Input: part model. Units: mm. Frame: model coordinates. A direction names the side the tool comes from. Coordinates: 2 decimals unless noted, no trailing zeros. Write each loop counter-clockwise with the first axis right and the second up, starting at its lowest first coordinate (ties: lowest second). Pieces come first, ordered by that corner, then holes. Notation, with made-up numbers: M 11.5,45.25 L 29.5,45.25 A18 ccw 29.5,58.25 Z; hole C 55,84.5 d7. An arc over 180 degrees is marked long. Use one line per item in the form item = value.
from build123d import *
from OCP.BRepFilletAPI import BRepFilletAPI_MakeChamfer

# Parameters (mm, degrees)
SKETCH_1_R          = 10
EXTRUDE_1_DEPTH     = 2
SKETCH_2_R          = 10
SKETCH_2_R_2        = 8.5
EXTRUDE_2_DEPTH     = 3
SKETCH_4_R          = 13.5
SKETCH_4_R_2        = 8.5
EXTRUDE_3_DEPTH     = 1
SKETCH_5_R          = 12.25
SKETCH_5_R_2        = 8.5
EXTRUDE_4_DEPTH     = 8
SKETCH_6_R          = 0.9
CUT_EXTRUDE_1_DEPTH = 8
SKETCH_7_R          = 3
SKETCH_7_R_2        = 1.15
CUT_EXTRUDE_2_DEPTH = 24.674881204
SKETCH_9_W          = 3
SKETCH_9_H          = 17
CUT_EXTRUDE_4_DEPTH = 24.674881204
EXTRUDE_5_DEPTH     = 3
CHAMFER_1_SIZE      = 0.2
CHAMFER_1_SIZE2     = 0.410060768


with BuildPart() as part:
    # 스케치1 → 보스-돌출1 (new body)
    with BuildSketch(Plane.XY):
        Circle(SKETCH_1_R)
    extrude(amount=EXTRUDE_1_DEPTH)

    # 스케치2 → 보스-돌출2 (add)
    with BuildSketch(Plane.XY.offset(2)):
        Circle(SKETCH_2_R)
        Circle(SKETCH_2_R_2, mode=Mode.SUBTRACT)
    extrude(amount=EXTRUDE_2_DEPTH)

    # 스케치4 → 보스-돌출3 (add)
    with BuildSketch(Plane.XY.offset(5)):
        Circle(SKETCH_4_R)
        Circle(SKETCH_4_R_2, mode=Mode.SUBTRACT)
    extrude(amount=EXTRUDE_3_DEPTH)

    # 스케치5 → 보스-돌출4 (add)
    with BuildSketch(Plane.XY.offset(6)):
        Circle(SKETCH_5_R)
        Circle(SKETCH_5_R_2, mode=Mode.SUBTRACT)
    extrude(amount=EXTRUDE_4_DEPTH)

    # 스케치6 → 컷-돌출1 (cut)
    with BuildSketch(Plane.XY.offset(14)):
        with Locations((10.375, 0)):
            Circle(SKETCH_6_R)
        with Locations((5.1875, -8.985013564)):
            Circle(SKETCH_6_R)
        with Locations((-5.1875, -8.985013564)):
            Circle(SKETCH_6_R)
        with Locations((-10.375, 0)):
            Circle(SKETCH_6_R)
        with Locations((-5.1875, 8.985013564)):
            Circle(SKETCH_6_R)
        with Locations((5.1875, 8.985013564)):
            Circle(SKETCH_6_R)
    extrude(amount=-CUT_EXTRUDE_1_DEPTH, mode=Mode.SUBTRACT)

    # 스케치7 → 컷-돌출2 (cut, through all)
    with BuildSketch(Plane(origin=(0, 0, 0), x_dir=(-1, 0, 0), z_dir=(0, 0, -1))):
        Circle(SKETCH_7_R)
        with Locations((-7, 0)):
            Circle(SKETCH_7_R_2)
        with Locations((7, 0)):
            Circle(SKETCH_7_R_2)
        with Locations((0, 7)):
            Circle(SKETCH_7_R_2)
        with Locations((0, -7)):
            Circle(SKETCH_7_R_2)
    extrude(amount=-CUT_EXTRUDE_2_DEPTH, mode=Mode.SUBTRACT)

    # 스케치9 → 컷-돌출4 (cut, through all)
    with BuildSketch(Plane(origin=(0, 0, 0), x_dir=(0, 0, -1), z_dir=(1, 0, 0))):
        with Locations((-3.5, 0)):
            Rectangle(SKETCH_9_W, SKETCH_9_H)
    extrude(amount=-CUT_EXTRUDE_4_DEPTH, mode=Mode.SUBTRACT)

    # 스케치10 → 보스-돌출5 (add)
    with BuildSketch(Plane.XY.offset(14)):
        with BuildLine():
            Line((2.199961883, 8.210369523), (2.717599974, 10.142221176))
            ThreePointArc((2.717599974, 10.142221176), (0, 10.5), (-2.717599974, 10.142221176))
            Line((-2.717599974, 10.142221176), (-2.199961883, 8.210369523))
            ThreePointArc((-2.199961883, 8.210369523), (0, 8.5), (2.199961883, 8.210369523))
        make_face()
        with BuildLine():
            Line((6.01040764, 6.01040764), (7.424621202, 7.424621202))
            ThreePointArc((7.424621202, 7.424621202), (9.09326674, 5.25), (10.142221176, 2.717599974))
            Line((10.142221176, 2.717599974), (8.210369523, 2.199961883))
            ThreePointArc((8.210369523, 2.199961883), (7.361215932, 4.25), (6.01040764, 6.01040764))
        make_face()
        with BuildLine():
            Line((8.210369523, -2.199961883), (10.142221176, -2.717599974))
            ThreePointArc((10.142221176, -2.717599974), (9.09326674, -5.25), (7.424621202, -7.424621202))
            Line((7.424621202, -7.424621202), (6.01040764, -6.01040764))
            ThreePointArc((6.01040764, -6.01040764), (7.361215932, -4.25), (8.210369523, -2.199961883))
        make_face()
        with BuildLine():
            Line((2.199961883, -8.210369523), (2.717599974, -10.142221176))
            ThreePointArc((2.717599974, -10.142221176), (0, -10.5), (-2.717599974, -10.142221176))
            Line((-2.717599974, -10.142221176), (-2.199961883, -8.210369523))
            ThreePointArc((-2.199961883, -8.210369523), (0, -8.5), (2.199961883, -8.210369523))
        make_face()
        with BuildLine():
            Line((-6.01040764, -6.01040764), (-7.424621202, -7.424621202))
            ThreePointArc((-7.424621202, -7.424621202), (-9.09326674, -5.25), (-10.142221176, -2.717599974))
            Line((-10.142221176, -2.717599974), (-8.210369523, -2.199961883))
            ThreePointArc((-8.210369523, -2.199961883), (-7.361215932, -4.25), (-6.01040764, -6.01040764))
        make_face()
        with BuildLine():
            Line((-8.210369523, 2.199961883), (-10.142221176, 2.717599974))
            ThreePointArc((-10.142221176, 2.717599974), (-9.09326674, 5.25), (-7.424621202, 7.424621202))
            Line((-7.424621202, 7.424621202), (-6.01040764, 6.01040764))
            ThreePointArc((-6.01040764, 6.01040764), (-7.361215932, 4.25), (-8.210369523, 2.199961883))
        make_face()
    extrude(amount=EXTRUDE_5_DEPTH)

    # 모따기1: one chamfer whose edges measure the first distance from different faces: ONE call of the kernel's chamfer builder (chamfer() names one face for all edges)
    chamfer_1_edges_1 = [part.edges().sort_by_distance(p)[0] for p in [
        (-6.717514421, 6.717514421, 17),
    ]]
    chamfer_1_side_1 = [part.faces().sort_by_distance(p)[0] for p in [
        (-6.717514421, 6.717514421, 15.5),
    ]]
    chamfer_1_edges_2 = [part.edges().sort_by_distance(p)[0] for p in [
        (-9.09326674, 5.25, 17),
    ]]
    chamfer_1_side_2 = [part.faces().sort_by_distance(p)[0] for p in [
        (-9.09326674, 5.25, 15.5),
    ]]
    chamfer_1_edges_3 = [part.edges().sort_by_distance(p)[0] for p in [
        (-9.17629535, 2.458780928, 17),
    ]]
    chamfer_1_side_3 = [part.faces().sort_by_distance(p)[0] for p in [
        (-9.17629535, 2.458780928, 15.5),
    ]]
    chamfer_1_edges_4 = [part.edges().sort_by_distance(p)[0] for p in [
        (-9.17629535, -2.458780928, 17),
    ]]
    chamfer_1_side_4 = [part.faces().sort_by_distance(p)[0] for p in [
        (-9.17629535, -2.458780928, 15.5),
    ]]
    chamfer_1_edges_5 = [part.edges().sort_by_distance(p)[0] for p in [
        (-9.09326674, -5.25, 17),
    ]]
    chamfer_1_side_5 = [part.faces().sort_by_distance(p)[0] for p in [
        (-9.09326674, -5.25, 15.5),
    ]]
    chamfer_1_edges_6 = [part.edges().sort_by_distance(p)[0] for p in [
        (-6.717514421, -6.717514421, 17),
    ]]
    chamfer_1_side_6 = [part.faces().sort_by_distance(p)[0] for p in [
        (-6.717514421, -6.717514421, 15.5),
    ]]
    chamfer_1_edges_7 = [part.edges().sort_by_distance(p)[0] for p in [
        (0, 10.5, 17),
    ]]
    chamfer_1_side_7 = [part.faces().sort_by_distance(p)[0] for p in [
        (0, 10.5, 15.5),
    ]]
    chamfer_1_edges_8 = [part.edges().sort_by_distance(p)[0] for p in [
        (-2.458780928, 9.17629535, 17),
    ]]
    chamfer_1_side_8 = [part.faces().sort_by_distance(p)[0] for p in [
        (-2.458780928, 9.17629535, 15.5),
    ]]
    chamfer_1_edges_9 = [part.edges().sort_by_distance(p)[0] for p in [
        (2.458780928, 9.17629535, 17),
    ]]
    chamfer_1_side_9 = [part.faces().sort_by_distance(p)[0] for p in [
        (2.458780928, 9.17629535, 15.5),
    ]]
    chamfer_1_edges_10 = [part.edges().sort_by_distance(p)[0] for p in [
        (-2.458780928, -9.17629535, 17),
    ]]
    chamfer_1_side_10 = [part.faces().sort_by_distance(p)[0] for p in [
        (-2.458780928, -9.17629535, 15.5),
    ]]
    chamfer_1_edges_11 = [part.edges().sort_by_distance(p)[0] for p in [
        (0, -10.5, 17),
    ]]
    chamfer_1_side_11 = [part.faces().sort_by_distance(p)[0] for p in [
        (0, -10.5, 15.5),
    ]]
    chamfer_1_edges_12 = [part.edges().sort_by_distance(p)[0] for p in [
        (2.458780928, -9.17629535, 17),
    ]]
    chamfer_1_side_12 = [part.faces().sort_by_distance(p)[0] for p in [
        (2.458780928, -9.17629535, 15.5),
    ]]
    chamfer_1_edges_13 = [part.edges().sort_by_distance(p)[0] for p in [
        (9.09326674, 5.25, 17),
    ]]
    chamfer_1_side_13 = [part.faces().sort_by_distance(p)[0] for p in [
        (9.09326674, 5.25, 15.5),
    ]]
    chamfer_1_edges_14 = [part.edges().sort_by_distance(p)[0] for p in [
        (6.717514421, 6.717514421, 17),
    ]]
    chamfer_1_side_14 = [part.faces().sort_by_distance(p)[0] for p in [
        (6.717514421, 6.717514421, 15.5),
    ]]
    chamfer_1_edges_15 = [part.edges().sort_by_distance(p)[0] for p in [
        (9.17629535, 2.458780928, 17),
    ]]
    chamfer_1_side_15 = [part.faces().sort_by_distance(p)[0] for p in [
        (9.17629535, 2.458780928, 15.5),
    ]]
    chamfer_1_edges_16 = [part.edges().sort_by_distance(p)[0] for p in [
        (6.717514421, -6.717514421, 17),
    ]]
    chamfer_1_side_16 = [part.faces().sort_by_distance(p)[0] for p in [
        (6.717514421, -6.717514421, 15.5),
    ]]
    chamfer_1_edges_17 = [part.edges().sort_by_distance(p)[0] for p in [
        (9.09326674, -5.25, 17),
    ]]
    chamfer_1_side_17 = [part.faces().sort_by_distance(p)[0] for p in [
        (9.09326674, -5.25, 15.5),
    ]]
    chamfer_1_edges_18 = [part.edges().sort_by_distance(p)[0] for p in [
        (9.17629535, -2.458780928, 17),
    ]]
    chamfer_1_side_18 = [part.faces().sort_by_distance(p)[0] for p in [
        (9.17629535, -2.458780928, 15.5),
    ]]
    chamfer_1 = BRepFilletAPI_MakeChamfer(part.part.solid().wrapped)
    for e in chamfer_1_edges_1:
        chamfer_1.Add(CHAMFER_1_SIZE, CHAMFER_1_SIZE2, e.wrapped, chamfer_1_side_1[0].wrapped)  # the first distance lies on this face
    for e in chamfer_1_edges_2:
        chamfer_1.Add(CHAMFER_1_SIZE, CHAMFER_1_SIZE2, e.wrapped, chamfer_1_side_2[0].wrapped)  # the first distance lies on this face
    for e in chamfer_1_edges_3:
        chamfer_1.Add(CHAMFER_1_SIZE, CHAMFER_1_SIZE2, e.wrapped, chamfer_1_side_3[0].wrapped)  # the first distance lies on this face
    for e in chamfer_1_edges_4:
        chamfer_1.Add(CHAMFER_1_SIZE, CHAMFER_1_SIZE2, e.wrapped, chamfer_1_side_4[0].wrapped)  # the first distance lies on this face
    for e in chamfer_1_edges_5:
        chamfer_1.Add(CHAMFER_1_SIZE, CHAMFER_1_SIZE2, e.wrapped, chamfer_1_side_5[0].wrapped)  # the first distance lies on this face
    for e in chamfer_1_edges_6:
        chamfer_1.Add(CHAMFER_1_SIZE, CHAMFER_1_SIZE2, e.wrapped, chamfer_1_side_6[0].wrapped)  # the first distance lies on this face
    for e in chamfer_1_edges_7:
        chamfer_1.Add(CHAMFER_1_SIZE, CHAMFER_1_SIZE2, e.wrapped, chamfer_1_side_7[0].wrapped)  # the first distance lies on this face
    for e in chamfer_1_edges_8:
        chamfer_1.Add(CHAMFER_1_SIZE, CHAMFER_1_SIZE2, e.wrapped, chamfer_1_side_8[0].wrapped)  # the first distance lies on this face
    for e in chamfer_1_edges_9:
        chamfer_1.Add(CHAMFER_1_SIZE, CHAMFER_1_SIZE2, e.wrapped, chamfer_1_side_9[0].wrapped)  # the first distance lies on this face
    for e in chamfer_1_edges_10:
        chamfer_1.Add(CHAMFER_1_SIZE, CHAMFER_1_SIZE2, e.wrapped, chamfer_1_side_10[0].wrapped)  # the first distance lies on this face
    for e in chamfer_1_edges_11:
        chamfer_1.Add(CHAMFER_1_SIZE, CHAMFER_1_SIZE2, e.wrapped, chamfer_1_side_11[0].wrapped)  # the first distance lies on this face
    for e in chamfer_1_edges_12:
        chamfer_1.Add(CHAMFER_1_SIZE, CHAMFER_1_SIZE2, e.wrapped, chamfer_1_side_12[0].wrapped)  # the first distance lies on this face
    for e in chamfer_1_edges_13:
        chamfer_1.Add(CHAMFER_1_SIZE, CHAMFER_1_SIZE2, e.wrapped, chamfer_1_side_13[0].wrapped)  # the first distance lies on this face
    for e in chamfer_1_edges_14:
        chamfer_1.Add(CHAMFER_1_SIZE, CHAMFER_1_SIZE2, e.wrapped, chamfer_1_side_14[0].wrapped)  # the first distance lies on this face
    for e in chamfer_1_edges_15:
        chamfer_1.Add(CHAMFER_1_SIZE, CHAMFER_1_SIZE2, e.wrapped, chamfer_1_side_15[0].wrapped)  # the first distance lies on this face
    for e in chamfer_1_edges_16:
        chamfer_1.Add(CHAMFER_1_SIZE, CHAMFER_1_SIZE2, e.wrapped, chamfer_1_side_16[0].wrapped)  # the first distance lies on this face
    for e in chamfer_1_edges_17:
        chamfer_1.Add(CHAMFER_1_SIZE, CHAMFER_1_SIZE2, e.wrapped, chamfer_1_side_17[0].wrapped)  # the first distance lies on this face
    for e in chamfer_1_edges_18:
        chamfer_1.Add(CHAMFER_1_SIZE, CHAMFER_1_SIZE2, e.wrapped, chamfer_1_side_18[0].wrapped)  # the first distance lies on this face
    add(Compound.cast(chamfer_1.Shape()), mode=Mode.REPLACE)


solid = part.part
(1) Set-up query: faces 4 (the cylindrical face through (-9.11, 5.22, 15.38)), 5 (the flat face through (2.253, -9.212, 16.901)), 6 (the flat face through (-3, 8.5, 4)). Return all of +Z, -Z, +X, -X, +Y, -Y with unobstructed straight access to the full face (end or side cutting, diameter ignored); none if empty.
Computed:
face_4 = +Z, -X, +Y
face_5 = +Z, +X
face_6 = -X
(2) First-contact query: pin 1 Ø9.5 at (x, y) = (0, 0) entering from +Z; pin 2 Ø1.5 at (y, z) = (-9, 15) entering from -X; pin 3 Ø2 at (x, y) = (-10.375, 0) entering from +Z. Flat tips, straight axial feed; report the tip coordinate or a pass-through.
Computed:
pin_1 = 2
pin_2 = -2.61
pin_3 = 14
(3) Section query C-C on x = -7. Return the cut outline in (y, z).
Computed:
outline = M -11.54,5 L -4.82,5 L -4.82,17 L -6.42,17 L -7,16.8 L -7,14 L -10.05,14 L -10.05,6 L -11.54,6 Z; M -7.14,0 L -1.15,0 L -1.15,2 L -7.14,2 Z; M 1.15,0 L 7.14,0 L 7.14,2 L 1.15,2 Z; M 4.82,5 L 11.54,5 L 11.54,6 L 10.05,6 L 10.05,14 L 7,14 L 7,16.8 L 6.42,17 L 4.82,17 Z
(4) Line query: probe 1 along Y at (x, z) = (0, 1.35); probe 2 along Y at (x, z) = (5.25, 7.5); probe 3 along Z at (x, y) = (-9.75, -1.25). Output: solid intervals per line, ascending.
Computed:
probe_1 = -10 to -8.15, -5.85 to -3, 3 to 5.85, 8.15 to 10
probe_2 = -11.07 to -9.88, -8.09 to -6.68, 6.68 to 8.09, 9.88 to 11.07
probe_3 = 0 to 2, 5 to 14
(5) Section query D-D on z = 4. Return the cut outline in (x, y).
Computed:
outline = M -5.27,-8.5 A10 ccw long -5.27,8.5 L 0,8.5 A8.5 cw 0,-8.5 Z
(6) Section query B-B on y = 1.75. Return the cut outline in (x, z).
Computed:
outline = M -13.39,5 L -8.32,5 L -8.32,14 L -12.12,14 L -12.12,6 L -13.39,6 Z; M -9.85,0 L -2.44,0 L -2.44,2 L -9.85,2 Z; M 2.44,0 L 9.85,0 L 9.85,5 L 13.39,5 L 13.39,6 L 12.12,6 L 12.12,14 L 8.32,14 L 8.32,2 L 2.44,2 Z
(7) Section query A-A on x = 7. Return the cut outline in (y, z), plus the area to 3 significant figures.
Computed:
outline = M -11.54,5 L -7.14,5 L -7.14,0 L -1.15,0 L -1.15,2 L -4.82,2 L -4.82,17 L -6.42,17 L -7,16.8 L -7,14 L -10.05,14 L -10.05,6 L -11.54,6 Z; M 1.15,0 L 7.14,0 L 7.14,5 L 11.54,5 L 11.54,6 L 10.05,6 L 10.05,14 L 7,14 L 7,16.8 L 6.42,17 L 4.82,17 L 4.82,2 L 1.15,2 Z
area = 148 mm^2
(8) Pull-direction query (X, two-part tool) for faces 1 (the flat face through (-2.462, 9.19, 15.38)), 2 (the flat face through (-10, 0, 6)), 3 (the flat face through (0, -9, 17)); classes: pulls with the +X half, pulls with the -X half, needs draft (parallel to the pull), parting line crosses it, or undercut.
Computed:
face_1 = pulls with the -X half
face_2 = undercut
face_3 = needs draft
